Could you check a few things on this model? Use its own coordinates, in mm. A direction names the side the tool comes from. Coordinates: 2 decimals unless noted, no trailing zeros. Order: outer loops, then holes, each group sorted by start corner. A loop starts at its lowest first (then second) coordinate and runs counter-clockwise, first axis right, second up. Notation, with made-up numbers: (63.25, 28) - (72.25, 28) arc R37 ccw to (72.25, 66) - close; hole circle Ø9 at (15, 38). An arc over 180 degrees is marked (long way). Answer as a JSON object with one key per item and string values. Group by question number.
(1) Please list where these lines run through material, in increasing order: probe 1 along Z at (x, y) = (2.8, 3.25); probe 2 along Z at (x, y) = (2.15, -14.5); probe 3 along Y at (x, z) = (1.6, 29).
(2) Which directions (+Z, -Z, +X, -X, +Y, -Y) give clear straight access to the entire face, cutting with the end or side of a thin tool? Please do faces 4 (the flat face through (0.5, 2.3, -3.3)), 5 (the cylindrical face through (2.218, -14.802, 59.192)).
(3) We'd pull the mould along Z, two halves only. Please class faces 1 (the cylindrical face through (2.218, 5.253, 59.153)), 2 (the flat face through (4.5, -5, 27)), 3 (the cylindrical face through (2.22, -17.4, 18.07)): pulls with the +Z half, pulls with the -Z half, needs draft (parallel to the pull), parting line crosses it, or undercut.
(4) Imagine slicing it at A-A, the plane y = -14.5. Write out the boundary of the cut face in (x, z), and give its area (3 significant figures).
(5) Imagine slicing it at B-B, the plane x = 1.85. Write out the boundary of the cut face in (y, z), and give its area (3 significant figures).
(6) Imagine slicing it at C-C, the plane y = -8.5. Write out the boundary of the cut face in (x, z), and give its area (3 significant figures).
(7) Will these pins go through, and if not, where does the flat tip stop? P1, Ø1, axis at x = 0.5, z = 43.5, coming from the -Y side; P2, Ø2, axis at x = 1, z = 48.5, coming from the +Y side; P3, Ø1.5, axis at x = 2, z = 29.5, coming from the +Y side.
from build123d import *

# Parameters (mm, degrees)
SKETCH_1_R          = 3.75
SKETCH_1_R_2        = 1.6
EXTRUDE_1_DEPTH     = 4.5
SKETCH_2_R          = 5.1
CUT_EXTRUDE_1_DEPTH = 4


with BuildPart() as part:
    # 草图1 → 凸台-拉伸1 (new body)
    with BuildSketch(Plane(origin=(0, 0, 0), x_dir=(0, 0, -1), z_dir=(1, 0, 0))):
        with BuildLine():
            Line((-15.79768273, -16.537533957), (3.488631385, -7.878744113))
            ThreePointArc((3.488631385, -7.878744113), (8.359485225, 1.66812029), (0.014361881, 8.393204188))
            Line((0.014361881, 8.393204188), (-61.98518523, 8.15622713))
            Line((-61.98518523, 8.15622713), (-61.910470293, -17.843665517))
            Line((-61.910470293, -17.843665517), (-20.410773437, -17.685043777))
            ThreePointArc((-20.410773437, -17.685043777), (-18.035050818, -17.389387577), (-15.79768273, -16.537533957))
        make_face()
        with Locations((0.046850671, -0.106733722)):
            Circle(SKETCH_1_R, mode=Mode.SUBTRACT)
        with Locations((-57.973718038, 4.171530696)):
            Circle(SKETCH_1_R_2, mode=Mode.SUBTRACT)
        with Locations((-24.922233336, -13.702270131)):
            Circle(SKETCH_1_R_2, mode=Mode.SUBTRACT)
        with Locations((-27.973937178, 4.286197014)):
            Circle(SKETCH_1_R_2, mode=Mode.SUBTRACT)
        with Locations((-57.921992313, -13.828394983)):
            Circle(SKETCH_1_R_2, mode=Mode.SUBTRACT)
    extrude(amount=EXTRUDE_1_DEPTH)

    # 草图2 → 切除-拉伸1 (cut)
    with BuildSketch(Plane(origin=(4.5, 0, 0), x_dir=(0, 0, -1), z_dir=(1, 0, 0))):
        Circle(SKETCH_2_R)
    extrude(amount=-CUT_EXTRUDE_1_DEPTH, mode=Mode.SUBTRACT)


solid = part.part
Result set:
{
 "1": {"probe 1": "z = -7.86 to -3.93, 3.93 to 26.75, 29.19 to 56.67, 59.28 to 61.97", "probe 2": "z = 11.26 to 23.54, 26.31 to 56.47, 59.37 to 61.92", "probe 3": "y = -17.72 to 3.06, 5.51 to 8.28"},
 "2": {"face 4": "+X", "face 5": "+X, -X"},
 "3": {"face 1": "undercut", "face 2": "needs draft", "face 3": "pulls with the -Z half"},
 "4": {"outline": "(0, 11.26) - (4.5, 11.26) - (4.5, 23.54) - (0, 23.54) - close; (0, 26.31) - (4.5, 26.31) - (4.5, 56.47) - (0, 56.47) - close; (0, 59.37) - (4.5, 59.37) - (4.5, 61.92) - (0, 61.92) - close", "area": "202 mm^2"},
 "5": {"outline": "(-17.84, 61.91) - (-17.69, 20.41) arc R10 ccw to (-16.54, 15.8) - (-7.88, -3.49) arc R8.5 ccw to (8.39, -0.01) - (8.16, 61.99) - close; hole circle Ø3.2 at (-13.83, 57.92); hole circle Ø3.2 at (-13.7, 24.92); hole circle Ø10.2 at (0, 0); hole circle Ø3.2 at (4.17, 57.97); hole circle Ø3.2 at (4.29, 27.97)", "area": "1,540 mm^2"},
 "6": {"outline": "(0, -2.1) - (4.5, -2.1) - (4.5, 61.94) - (0, 61.94) - close", "area": "288 mm^2"},
 "7": {"P1": "stops at y = -17.78", "P2": "stops at y = 8.21", "P3": "stops at y = 8.28"}
}
